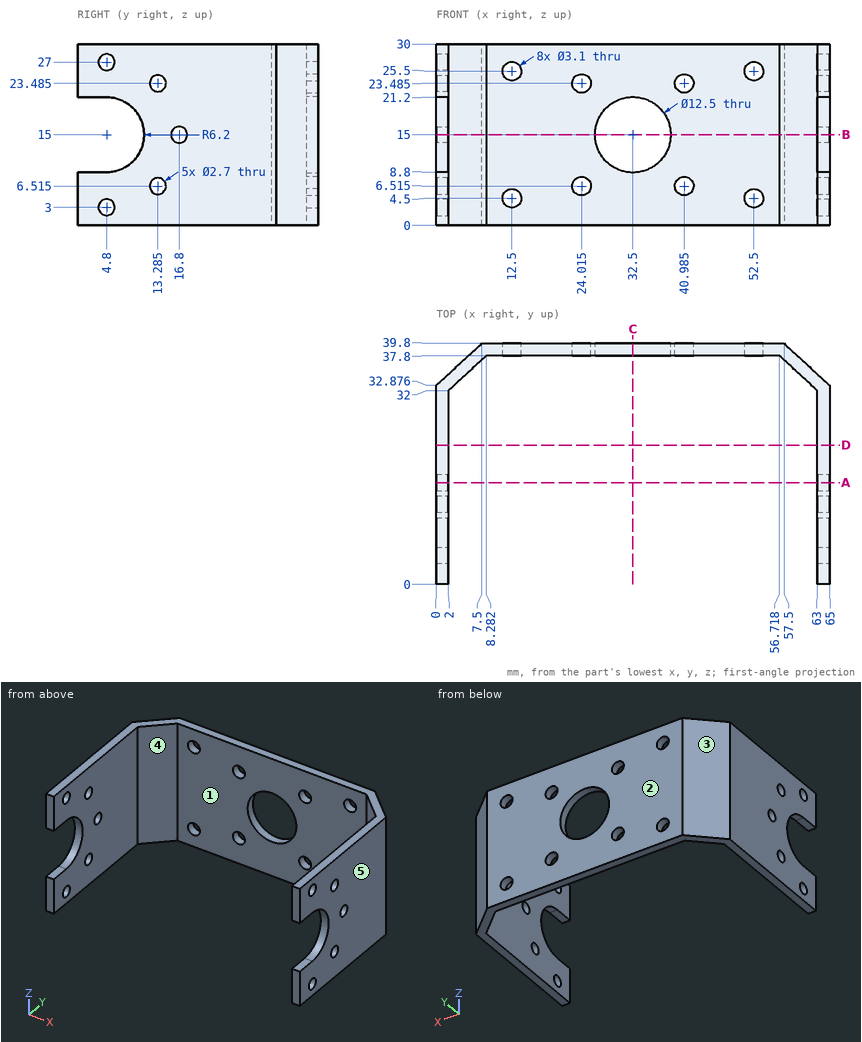
Geometry: see drawing. Coordinates: mm, zero at the bounding-box minimum. A direction names the side the tool comes from. Round coordinates to 2 decimals unless told otherwise and drop trailing zeros. Loops run counter-clockwise (first coordinate to the right, second up) from the corner with the lowest first, then second, coordinate; pieces in that order, holes last. Notation, with made-up numbers: M -9,40.25 L 41,40.25 A29 cw 41,79.25 Z; hole C 9,-7 d8. An arc over 180 degrees is marked long. Use a Markdown table: item, result. Add a question column.
1. Section query A-A on y = 16.8. Return the cut outline in (x, z).
2. Line query: line 1 (X direction, y = 11.5, z = 25); line 2 (Y direction, x = 16, z = 17.5); line 3 (Y direction, x = 1.4, z = 27). Output: solid intervals per line, ascending.
3. Section query D-D on y = 23. Return the cut outline in (x, z), then the cut area to 3 significant figures.
4. Mould query, pull axis X, two halves, no side actions, for the marked faces 3, 4 and 5. Classes: pulls with the +X half, pulls with the -X half, needs draft (parallel to the pull), parting line crosses it, or undercut.
5. Section query C-C on x = 32.5. Return the cut outline in (y, z).
6. Contact query for flat-ended pins moving along their axis: P1, Ø3.5, axis at x = 24.01, z = 6.51, coming from the +Y side; P2, Ø1.5, axis at x = 17.5, z = 10.5, coming from the -Y side. Output: stop coordinate, or through.
7. Reachability of the marked faces 1 and 2 from +Z, -Z, +X, -X, +Y, -Y: full face, straight path, thin tool, end or side. Return the list, or none.
8. Section query B-B on z = 15. Give the number of separate pieces and of enclosed holes in the cut face, then the cut area to 3 significant figures.
Reported:
| question | item | result |
|---|---|---|
| 1 | outline | M 0,0 L 2,0 L 2,13.65 L 0,13.65 Z; M 0,16.35 L 2,16.35 L 2,30 L 0,30 Z; M 63,0 L 65,0 L 65,13.65 L 63,13.65 Z; M 63,16.35 L 65,16.35 L 65,30 L 63,30 Z |
| 2 | line 1 | x = 0 to 2, 63 to 65 |
| 2 | line 2 | y = 37.8 to 39.8 |
| 2 | line 3 | y = 0 to 3.45, 6.15 to 34.17 |
| 3 | outline | M 0,0 L 2,0 L 2,30 L 0,30 Z; M 63,0 L 65,0 L 65,30 L 63,30 Z |
| 3 | area | 120 mm² |
| 4 | face 3 | pulls with the -X half |
| 4 | face 4 | undercut |
| 4 | face 5 | pulls with the +X half |
| 5 | outline | M 37.8,0 L 39.8,0 L 39.8,8.75 L 37.8,8.75 Z; M 37.8,21.25 L 39.8,21.25 L 39.8,30 L 37.8,30 Z |
| 6 | P1 | stops at y = 39.8 |
| 6 | P2 | stops at y = 37.8 |
| 7 | face 1 | +Z, -Z, -Y |
| 7 | face 2 | +Z, -Z, +X, -X, +Y |
| 8 | separate pieces | 4 |
| 8 | enclosed holes | 0 |
| 8 | area | 186 mm² |
